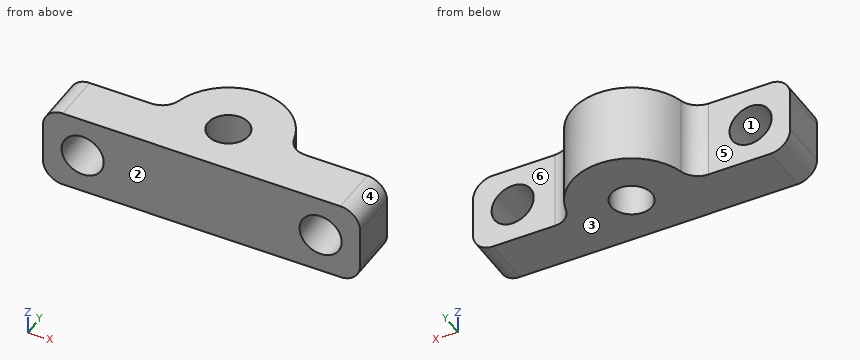
from build123d import *

# Parameters (mm, degrees)
SKETCH2_R           = 2.05
BOSS_EXTRUDE1_DEPTH = 8
SKETCH3_R           = 2.125
CUT_EXTRUDE1_DEPTH  = 8
FILLET1_R           = 2


with BuildPart() as part:
    # Sketch2 → Boss-Extrude1 (new body)
    with BuildSketch(Plane.XY):
        with BuildLine():
            Line((6, 2.5), (16, 2.5))
            Line((16, 2.5), (16, -2.5))
            Line((16, -2.5), (-16, -2.5))
            Line((-16, -2.5), (-16, 2.5))
            Line((-16, 2.5), (-6, 2.5))
            ThreePointArc((-6, 2.5), (0, 8.5), (6, 2.5))
        make_face()
        with Locations((0, 2.5)):
            Circle(SKETCH2_R, mode=Mode.SUBTRACT)
    extrude(amount=BOSS_EXTRUDE1_DEPTH)

    # Sketch3 → Cut-Extrude1 (cut)
    with BuildSketch(Plane(origin=(0, 2.5, 0), x_dir=(1, 0, 0), z_dir=(0, 1, 0))):
        with Locations((12, -4)):
            Circle(SKETCH3_R)
        with Locations((-12, -4)):
            Circle(SKETCH3_R)
    extrude(amount=-CUT_EXTRUDE1_DEPTH, mode=Mode.SUBTRACT)

    # Fillet1
    fillet1_edges = [part.edges().sort_by_distance(p)[0] for p in [
        (-6, 2.5, 4),
        (6, 2.5, 4),
        (-16, 0, 8),
        (16, 0, 8),
        (-16, 0, 0),
        (16, 0, 0),
    ]]
    fillet(fillet1_edges, radius=FILLET1_R)


solid = part.part
Here's how the part is built. I have some questions about the finished solid (model axes, mm). Face numbers are marked on the shaded views. A direction names the side the tool comes from. Coordinates: 2 decimals unless noted, no trailing zeros. Write each loop counter-clockwise with the first axis right and the second up, starting at its lowest first coordinate (ties: lowest second). Pieces come first, ordered by that corner, then holes.
1) If I drill on line 1 (X direction, y = -1.35, z = 4) (3 decimals); line 2 (X direction, y = 0.95, z = 4) (3 decimals); line 3 (Z direction, x = 12, y = 1.25) (3 decimals), over which ranges is the centre line in solid material (lowest first)?
Filled in:
line 1: x = -16 to -14.125, -9.875 to 9.875, 14.125 to 16
line 2: x = -16 to -14.125, -9.875 to -1.342, 1.342 to 9.875, 14.125 to 16
line 3: z = 0 to 1.875, 6.125 to 8
2) If we section it at A-A (z = 4): List the corners of the cut face in (x, y) for me (3 decimals).
Filled in:
outline: (-16, -2.5) - (-14.125, -2.5) - (-14.125, 2.5) - (-16, 2.5) - close; (-9.875, -2.5) - (9.875, -2.5) - (9.875, 2.5) - (7.746, 2.5) arc R2 cw to (5.809, 4) arc R6 ccw to (-5.809, 4) arc R2 cw to (-7.746, 2.5) - (-9.875, 2.5) - close; (14.125, -2.5) - (16, -2.5) - (16, 2.5) - (14.125, 2.5) - close; hole circle Ø4.1 at (0, 2.5)
3) If we section it at B-B (x = 12): List the corners of the cut face in (y, z) for me (3 decimals).
Filled in:
outline: (-2.5, 0) - (2.5, 0) - (2.5, 1.875) - (-2.5, 1.875) - close; (-2.5, 6.125) - (2.5, 6.125) - (2.5, 8) - (-2.5, 8) - close
4) If we section it at C-C (y = 2): List the corners of the cut face in (x, z) for me (3 decimals), plus the area to 3 significant figures.
Filled in:
outline: (-16, 2) arc R2 ccw to (-14, 0) - (-1.988, 0) - (-1.988, 8) - (-14, 8) arc R2 ccw to (-16, 6) - close; (1.988, 0) - (14, 0) arc R2 ccw to (16, 2) - (16, 6) arc R2 ccw to (14, 8) - (1.988, 8) - close; hole circle Ø4.25 at (-12, 4); hole circle Ø4.25 at (12, 4)
area: 192 mm2
5) If we section it at D-D (y = -1): List the corners of the cut face in (x, z) for me (3 decimals).
Filled in:
outline: (-16, 2) arc R2 ccw to (-14, 0) - (14, 0) arc R2 ccw to (16, 2) - (16, 6) arc R2 ccw to (14, 8) - (-14, 8) arc R2 ccw to (-16, 6) - close; hole circle Ø4.25 at (-12, 4); hole circle Ø4.25 at (12, 4)
6) Which directions (+Z, -Z, +X, -X, +Y, -Y) give clear straight access to the entire face, cutting with the end or side of a thin tool? Please do the marked faces 4, 5 and 6.
Filled in:
face 4: +Z, +X, +Y, -Y
face 5: +Z, -Z, -X, +Y
face 6: +Z, -Z, +X, +Y
7) Thinking about a two-plate mould opening in Z: for the marked faces 1, 2 and 3, which applies, +Z half, -Z half, draft (parallel to the pull), parting line (faces both ways), or undercut?
Filled in:
face 1: undercut
face 2: draft
face 3: -Z half
8) I'm going to push flat-ended pins straight in: pin 1 (4 mm diameter, centred on x = 11.5, z = 2.5, fed in from +Y); pin 2 (3 mm diameter, centred on x = -4.5, z = 5.5, fed in from +Y). Where does each tip first touch, or does it pass through?
Filled in:
pin 1: stops at y = 2.5
pin 2: stops at y = 7.7
